Check sheet for the modelled part. Datum: model origin and axes. Units: mm. A direction names the side the tool comes from. Give positions to 0.01 mm unless a question says otherwise; leave off trailing zeros. Order: outer loops, then holes, each group sorted by start corner. A loop starts at its lowest first (then second) coordinate and runs counter-clockwise, first axis right, second up. Notation, with made-up numbers: (-17, 37.5) -> (14, 37.5) arc R34 ccw to (14, 74.5) -> close; hole circle Ø4 at (-21, 87). An arc over 180 degrees is marked (long way). One line per question, with ' | ' between items.
```python
from build123d import *

# Parameters (mm, degrees)
F_20_SERIES_20_2020_1_DEPTH = 55


with BuildPart() as part:
    # Sketch11 → 20_series 20-2020(1) (new body)
    with BuildSketch(Plane(origin=(0, 0, 0), x_dir=(0, 0, -1), z_dir=(1, 0, 0))):
        with BuildLine():
            Line((9.0094, 2.6289), (9.492, 2.6289))
            ThreePointArc((9.492, 2.6289), (9.851210245, 2.777689755), (10, 3.1369))
            Line((10, 3.1369), (10, 8.5014))
            ThreePointArc((10, 8.5014), (9.561070222, 9.561070222), (8.5014, 10))
            Line((8.5014, 10), (3.1369, 10))
            ThreePointArc((3.1369, 10), (2.777689755, 9.851210245), (2.6289, 9.492))
            Line((2.6289, 9.492), (2.6289, 9.0094))
            ThreePointArc((2.6289, 9.0094), (2.777689755, 8.650189755), (3.1369, 8.5014))
            Line((3.1369, 8.5014), (5.4864, 8.5014))
            ThreePointArc((5.4864, 8.5014), (5.845610245, 8.352610245), (5.9944, 7.9934))
            Line((5.9944, 7.9934), (5.9944, 7.264490712))
            ThreePointArc((5.9944, 7.264490712), (5.955730803, 7.070087528), (5.845610245, 6.905280467))
            Line((5.845610245, 6.905280467), (2.747686782, 3.807357004))
            ThreePointArc((2.747686782, 3.807357004), (2.582879721, 3.697236446), (2.388476537, 3.658567249))
            Line((2.388476537, 3.658567249), (-2.388476537, 3.658567249))
            ThreePointArc((-2.388476537, 3.658567249), (-2.582879721, 3.697236446), (-2.747686782, 3.807357004))
            Line((-2.747686782, 3.807357004), (-5.845610245, 6.905280467))
            ThreePointArc((-5.845610245, 6.905280467), (-5.955730803, 7.070087528), (-5.9944, 7.264490712))
            Line((-5.9944, 7.264490712), (-5.9944, 7.9934))
            ThreePointArc((-5.9944, 7.9934), (-5.845610245, 8.352610245), (-5.4864, 8.5014))
            Line((-5.4864, 8.5014), (-3.1369, 8.5014))
            ThreePointArc((-3.1369, 8.5014), (-2.777689755, 8.650189755), (-2.6289, 9.0094))
            Line((-2.6289, 9.0094), (-2.6289, 9.492))
            ThreePointArc((-2.6289, 9.492), (-2.777689755, 9.851210245), (-3.1369, 10))
            Line((-3.1369, 10), (-8.5014, 10))
            ThreePointArc((-8.5014, 10), (-9.561070222, 9.561070222), (-10, 8.5014))
            Line((-10, 8.5014), (-10, 3.1369))
            ThreePointArc((-10, 3.1369), (-9.851210245, 2.777689755), (-9.492, 2.6289))
            Line((-9.492, 2.6289), (-9.0094, 2.6289))
            ThreePointArc((-9.0094, 2.6289), (-8.650189755, 2.777689755), (-8.5014, 3.1369))
            Line((-8.5014, 3.1369), (-8.5014, 5.4864))
            ThreePointArc((-8.5014, 5.4864), (-8.352610245, 5.845610245), (-7.9934, 5.9944))
            Line((-7.9934, 5.9944), (-7.264490712, 5.9944))
            ThreePointArc((-7.264490712, 5.9944), (-7.070087528, 5.955730803), (-6.905280467, 5.845610245))
            Line((-6.905280467, 5.845610245), (-3.807357004, 2.747686782))
            ThreePointArc((-3.807357004, 2.747686782), (-3.697236446, 2.582879721), (-3.658567249, 2.388476537))
            Line((-3.658567249, 2.388476537), (-3.658567249, -2.388476537))
            ThreePointArc((-3.658567249, -2.388476537), (-3.697236446, -2.582879721), (-3.807357004, -2.747686782))
            Line((-3.807357004, -2.747686782), (-6.905280467, -5.845610245))
            ThreePointArc((-6.905280467, -5.845610245), (-7.070087528, -5.955730803), (-7.264490712, -5.9944))
            Line((-7.264490712, -5.9944), (-7.9934, -5.9944))
            ThreePointArc((-7.9934, -5.9944), (-8.352610245, -5.845610245), (-8.5014, -5.4864))
            Line((-8.5014, -5.4864), (-8.5014, -3.1369))
            ThreePointArc((-8.5014, -3.1369), (-8.650189755, -2.777689755), (-9.0094, -2.6289))
            Line((-9.0094, -2.6289), (-9.492, -2.6289))
            ThreePointArc((-9.492, -2.6289), (-9.851210245, -2.777689755), (-10, -3.1369))
            Line((-10, -3.1369), (-10, -8.5014))
            ThreePointArc((-10, -8.5014), (-9.561070222, -9.561070222), (-8.5014, -10))
            Line((-8.5014, -10), (-3.1369, -10))
            ThreePointArc((-3.1369, -10), (-2.777689755, -9.851210245), (-2.6289, -9.492))
            Line((-2.6289, -9.492), (-2.6289, -9.0094))
            ThreePointArc((-2.6289, -9.0094), (-2.777689755, -8.650189755), (-3.1369, -8.5014))
            Line((-3.1369, -8.5014), (-5.4864, -8.5014))
            ThreePointArc((-5.4864, -8.5014), (-5.845610245, -8.352610245), (-5.9944, -7.9934))
            Line((-5.9944, -7.9934), (-5.9944, -7.264490712))
            ThreePointArc((-5.9944, -7.264490712), (-5.955730803, -7.070087528), (-5.845610245, -6.905280467))
            Line((-5.845610245, -6.905280467), (-2.747686782, -3.807357004))
            ThreePointArc((-2.747686782, -3.807357004), (-2.582879721, -3.697236446), (-2.388476537, -3.658567249))
            Line((-2.388476537, -3.658567249), (2.388476537, -3.658567249))
            ThreePointArc((2.388476537, -3.658567249), (2.582879721, -3.697236446), (2.747686782, -3.807357004))
            Line((2.747686782, -3.807357004), (5.845610245, -6.905280467))
            ThreePointArc((5.845610245, -6.905280467), (5.955730803, -7.070087528), (5.9944, -7.264490712))
            Line((5.9944, -7.264490712), (5.9944, -7.9934))
            ThreePointArc((5.9944, -7.9934), (5.845610245, -8.352610245), (5.4864, -8.5014))
            Line((5.4864, -8.5014), (3.1369, -8.5014))
            ThreePointArc((3.1369, -8.5014), (2.777689755, -8.650189755), (2.6289, -9.0094))
            Line((2.6289, -9.0094), (2.6289, -9.492))
            ThreePointArc((2.6289, -9.492), (2.777689755, -9.851210245), (3.1369, -10))
            Line((3.1369, -10), (8.5014, -10))
            ThreePointArc((8.5014, -10), (9.561070222, -9.561070222), (10, -8.5014))
            Line((10, -8.5014), (10, -3.1369))
            ThreePointArc((10, -3.1369), (9.851210245, -2.777689755), (9.492, -2.6289))
            Line((9.492, -2.6289), (9.0094, -2.6289))
            ThreePointArc((9.0094, -2.6289), (8.650189755, -2.777689755), (8.5014, -3.1369))
            Line((8.5014, -3.1369), (8.5014, -5.4864))
            ThreePointArc((8.5014, -5.4864), (8.352610245, -5.845610245), (7.9934, -5.9944))
            Line((7.9934, -5.9944), (7.264490712, -5.9944))
            ThreePointArc((7.264490712, -5.9944), (7.070087528, -5.955730803), (6.905280467, -5.845610245))
            Line((6.905280467, -5.845610245), (3.807357004, -2.747686782))
            ThreePointArc((3.807357004, -2.747686782), (3.697236446, -2.582879721), (3.658567249, -2.388476537))
            Line((3.658567249, -2.388476537), (3.658567249, 2.388476537))
            ThreePointArc((3.658567249, 2.388476537), (3.697236446, 2.582879721), (3.807357004, 2.747686782))
            Line((3.807357004, 2.747686782), (6.905280467, 5.845610245))
            ThreePointArc((6.905280467, 5.845610245), (7.070087528, 5.955730803), (7.264490712, 5.9944))
            Line((7.264490712, 5.9944), (7.9934, 5.9944))
            ThreePointArc((7.9934, 5.9944), (8.352610245, 5.845610245), (8.5014, 5.4864))
            Line((8.5014, 5.4864), (8.5014, 3.1369))
            ThreePointArc((8.5014, 3.1369), (8.650189755, 2.777689755), (9.0094, 2.6289))
        make_face()
        with BuildLine():
            Line((-2.296558466, 2.121727546), (-2.121727546, 2.296558466))
            ThreePointArc((-2.121727546, 2.296558466), (-1.459775814, 2.520126613), (-0.880635441, 2.129282347))
            ThreePointArc((-0.880635441, 2.129282347), (-0.755121693, 2.019456424), (-0.588548999, 2.011151493))
            ThreePointArc((-0.588548999, 2.011151493), (0, 2.0955), (0.588548999, 2.011151493))
            ThreePointArc((0.588548999, 2.011151493), (0.755121693, 2.019456424), (0.880635441, 2.129282347))
            ThreePointArc((0.880635441, 2.129282347), (1.459775814, 2.520126613), (2.121727546, 2.296558466))
            Line((2.121727546, 2.296558466), (2.296558466, 2.121727546))
            ThreePointArc((2.296558466, 2.121727546), (2.520126613, 1.459775814), (2.129282347, 0.880635441))
            ThreePointArc((2.129282347, 0.880635441), (2.019456424, 0.755121693), (2.011151493, 0.588548999))
            ThreePointArc((2.011151493, 0.588548999), (2.0955, 0), (2.011151493, -0.588548999))
            ThreePointArc((2.011151493, -0.588548999), (2.019456424, -0.755121693), (2.129282347, -0.880635441))
            ThreePointArc((2.129282347, -0.880635441), (2.520126613, -1.459775814), (2.296558466, -2.121727546))
            Line((2.296558466, -2.121727546), (2.121727546, -2.296558466))
            ThreePointArc((2.121727546, -2.296558466), (1.459775814, -2.520126613), (0.880635441, -2.129282347))
            ThreePointArc((0.880635441, -2.129282347), (0.755121693, -2.019456424), (0.588548999, -2.011151493))
            ThreePointArc((0.588548999, -2.011151493), (0, -2.0955), (-0.588548999, -2.011151493))
            ThreePointArc((-0.588548999, -2.011151493), (-0.755121693, -2.019456424), (-0.880635441, -2.129282347))
            ThreePointArc((-0.880635441, -2.129282347), (-1.459775814, -2.520126613), (-2.121727546, -2.296558466))
            Line((-2.121727546, -2.296558466), (-2.296558466, -2.121727546))
            ThreePointArc((-2.296558466, -2.121727546), (-2.520126613, -1.459775814), (-2.129282347, -0.880635441))
            ThreePointArc((-2.129282347, -0.880635441), (-2.019456424, -0.755121693), (-2.011151493, -0.588548999))
            ThreePointArc((-2.011151493, -0.588548999), (-2.0955, 0), (-2.011151493, 0.588548999))
            ThreePointArc((-2.011151493, 0.588548999), (-2.019456424, 0.755121693), (-2.129282347, 0.880635441))
            ThreePointArc((-2.129282347, 0.880635441), (-2.520126613, 1.459775814), (-2.296558466, 2.121727546))
        make_face(mode=Mode.SUBTRACT)
    extrude(amount=F_20_SERIES_20_2020_1_DEPTH)


solid = part.part
```
Q1. Thickness scan on line 1 (Y direction, x = 23, z = -1.5); line 2 (Z direction, x = 44, y = -0.75); line 3 (Z direction, x = 41, y = 4). Record the ranges inside material, lowest first.
Result sheet:
line 1: y = -3.66 to -2.52, 2.52 to 3.66 | line 2: z = -3.66 to -2.02, 2.02 to 3.66 | line 3: z = -10 to -8.5, -5.06 to -2.94, 2.94 to 5.06, 8.5 to 10
Q2. Depth check by flat-ended pin: pin 1 Ø4 at (x, z) = (27.5, -1) entering from +Y; pin 2 Ø4 at (x, z) = (16, 0.5) entering from -Y; pin 3 Ø0.5 at (x, y) = (31, 9) entering from -Z. Enter the tip coordinate at first touch or a pass-through.
Result sheet:
pin 1: stops at y = 9.98 | pin 2: stops at y = -3.67 | pin 3: stops at z = -9.98
Q3. Access from +Z, -Z, +X, -X, +Y, -Y to the whole of each face (thin tool, end or side, straight path). Record for faces 1 (the face through (27, 3.659, 0)), 2 (the face through (27.12, 1.47, -2.52)), 3 (the face through (0, 0.1, 2.4)).
Result sheet:
face 1: +X, -X, +Y | face 2: +X, -X | face 3: +Z, -Z, -X, +Y, -Y
Q4. Mould release check, pull along Y, two halves, no side actions. Record for faces 4 (the face through (27.12, 9.57, 9.55)), 5 (the face through (27, -10, 6)), 6 (the face through (27, -4, -8.501)): pulls with the +Y half, pulls with the -Y half, needs draft (parallel to the pull), parting line crosses it, or undercut.
Result sheet:
face 4: pulls with the +Y half | face 5: pulls with the -Y half | face 6: undercut
Q5. Section check A-A (z = 0). Enter the section's corners in (x, y), and give its area (3 significant figures).
Result sheet:
outline: (0, -3.66) -> (55, -3.66) -> (55, -2.1) -> (0, -2.1) -> close; (0, 2.1) -> (55, 2.1) -> (55, 3.66) -> (0, 3.66) -> close | area: 172 mm2
Q6. Section check B-B (y = -4.5). Enter the section's corners in (x, z), and give its area (3 significant figures).
Result sheet:
outline: (0, -10) -> (55, -10) -> (55, -8.5) -> (0, -8.5) -> close; (0, -5.56) -> (55, -5.56) -> (55, -3.44) -> (0, -3.44) -> close; (0, 3.44) -> (55, 3.44) -> (55, 5.56) -> (0, 5.56) -> close; (0, 8.5) -> (55, 8.5) -> (55, 10) -> (0, 10) -> close | area: 398 mm2
